Geometry: see drawing. Coordinates: mm, zero at the bounding-box minimum. A direction names the side the tool comes from. Give positions to 0.01 mm unless a question says otherwise; leave off trailing zeros. Loops run counter-clockwise (first coordinate to the right, second up) from the corner with the lowest first, then second, coordinate; pieces in that order, holes last. Notation, with made-up numbers: M -23,-39.75 L -2,-39.75 A20 cw -2,-4.75 Z; hole C -22,86.25 d6. An arc over 180 degrees is marked long. Put each result on its own line as item: value.
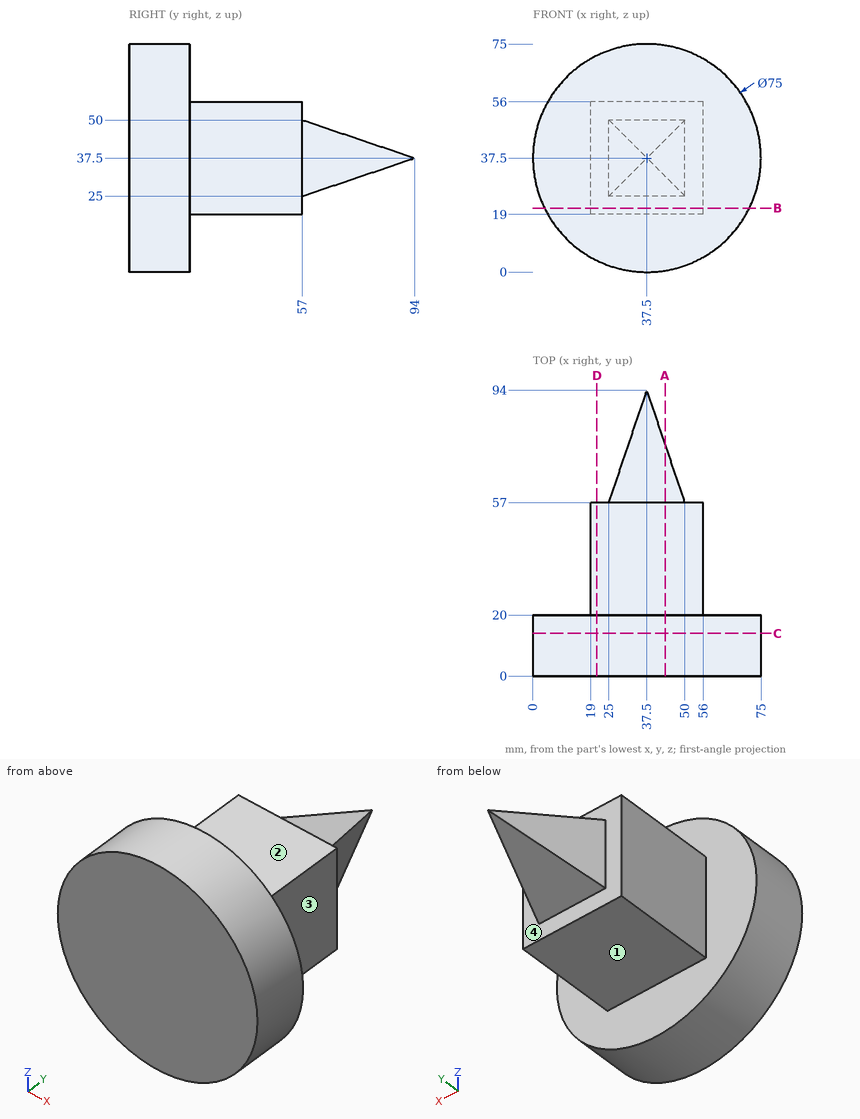
1. Section query B-B (z = 21). Output: boundary loops of the cut face in (x, y).
Found:
outline: M 3.83,0 L 71.17,0 L 71.17,20 L 56,20 L 56,57 L 19,57 L 19,20 L 3.83,20 Z
2. Material intervals for line 1 (Y direction, x = 42, z = 11); line 2 (Y direction, x = 54.5, z = 38); line 3 (Z direction, x = 30.5, y = 31.5), sorted ascending. Write a range as from..to.
Found:
line 1: 0..20
line 2: 0..57
line 3: 19..56
3. Section query D-D (x = 21). Output: boundary loops of the cut face in (y, z), plus the area to 3 significant figures.
Found:
outline: M 0,3.83 L 20,3.83 L 20,19 L 57,19 L 57,56 L 20,56 L 20,71.17 L 0,71.17 Z
area: 2,720 mm^2
4. Section query C-C (y = 14). Output: boundary loops of the cut face in (x, z), plus the area to 3 significant figures.
Found:
outline: C 37.5,37.5 d75
area: 4,420 mm^2
5. Contact query for flat-ended pins moving along their axis: P1, Ø2, axis at x = 63, z = 41, coming from the +Y side; P2, Ø8, axis at x = 54, z = 56.5, coming from the +Y side; P3, Ø18.5, axis at x = 29, y = 34, coming from the +Z side. Output: stop coordinate, or through.
Found:
P1: y = 20
P2: y = 57
P3: z = 56
6. Section query A-A (x = 43.5). Output: boundary loops of the cut face in (y, z), plus the area to 3 significant figures.
Found:
outline: M 0,0.48 L 20,0.48 L 20,19 L 57,19 L 57,25 L 76.24,31.5 L 76.24,43.5 L 57,50 L 57,56 L 20,56 L 20,74.52 L 0,74.52 Z
area: 3,210 mm^2
7. Access query for the marked faces 1, 2, 3 and 4. Directions: +Z, -Z, +X, -X, +Y, -Y. A direction counts if a zero-diameter tool reaches every point of the face in a straight line with its end or side. Return the directions, or none.
Found:
face 1: -Z, +X, -X, +Y
face 2: +Z, +X, -X, +Y
face 3: +Z, -Z, +X, +Y
face 4: +Y
